Geometry check sheet. Reference: drawing and pictorial views, mm from the part's lowest x, y, z. Coordinates: 2 decimals unless noted, no trailing zeros. Write each loop counter-clockwise with the first axis right and the second up, starting at its lowest first coordinate (ties: lowest second). Pieces come first, ordered by that corner, then holes. Notation, with made-up numbers: (65, 48) -> (98, 48) arc R36 ccw to (98, 82) -> close; hole circle Ø2 at (14.5, 65). An arc over 180 degrees is marked (long way). Use a Markdown table: item, result.
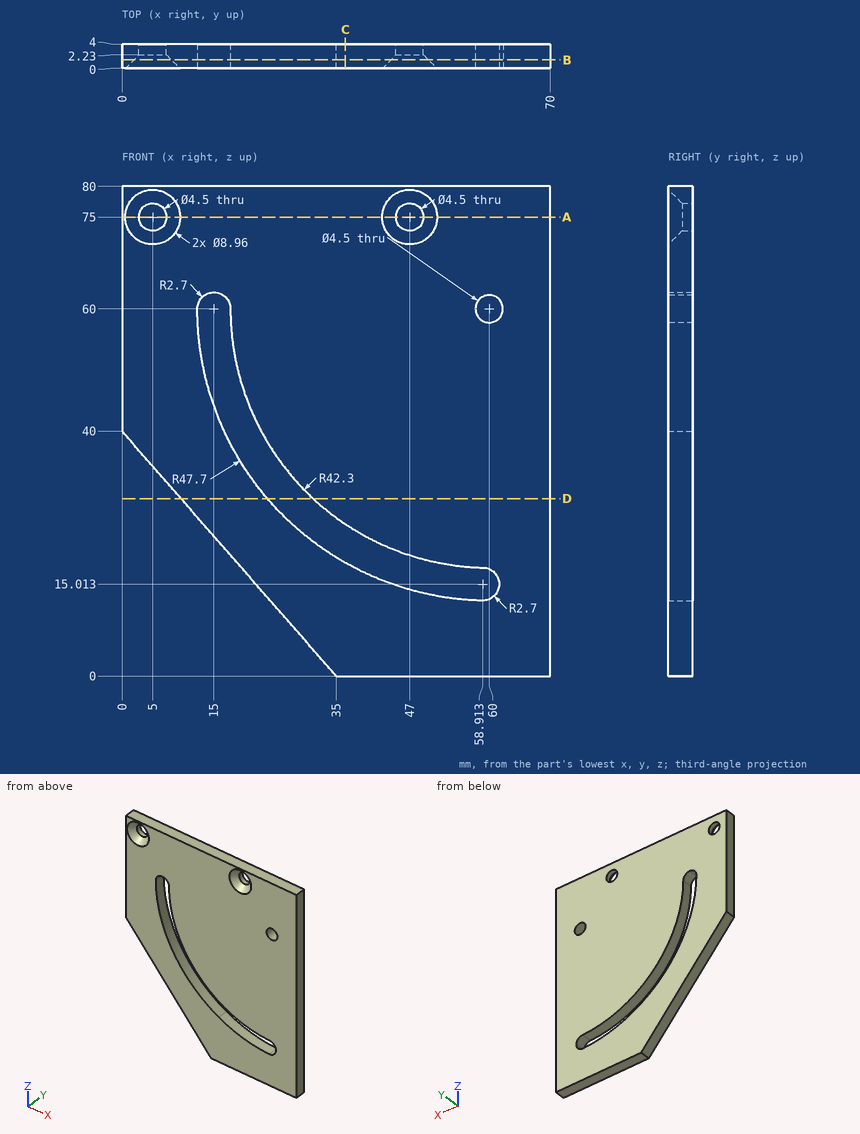
Item 1: Depth check by flat-ended pin: P1, Ø5, axis at x = 5, z = 75, coming from the -Y side; P2, Ø1, axis at x = 16.5, y = 2.5, coming from the -Z side. Enter the tip coordinate at first touch or a pass-through.
Answer block:
| item | result |
|---|---|
| P1 | stops at y = 1.98 |
| P2 | stops at z = 20.57 |
Item 2: Section check A-A on z = 75. Record the boundary of the cut face in (x, y).
Answer block:
| item | result |
|---|---|
| outline | (0, 0) -> (0.52, 0) -> (2.75, 2.23) -> (2.75, 4) -> (0, 4) -> close; (7.25, 2.23) -> (9.48, 0) -> (42.52, 0) -> (44.75, 2.23) -> (44.75, 4) -> (7.25, 4) -> close; (49.25, 2.23) -> (51.48, 0) -> (70, 0) -> (70, 4) -> (49.25, 4) -> close |
Item 3: Section check D-D on z = 29. Record the boundary of the cut face in (x, y) (3 decimals).
Answer block:
| item | result |
|---|---|
| outline | (9.625, 0) -> (23.747, 0) -> (23.747, 4) -> (9.625, 4) -> close; (31.22, 0) -> (70, 0) -> (70, 4) -> (31.22, 4) -> close |
Item 4: Section check B-B on y = 1.4. Count the separate pieces of the cut face and the enclosed holes in it, then the cut area to 3 significant figures.
Answer block:
| item | result |
|---|---|
| separate pieces | 1 |
| enclosed holes | 4 |
| area | 4,430 mm^2 |
Item 5: Section check C-C on x = 36.5. Record the boundary of the cut face in (y, z).
Answer block:
| item | result |
|---|---|
| outline | (0, 0) -> (4, 0) -> (4, 18.49) -> (0, 18.49) -> close; (0, 24.83) -> (4, 24.83) -> (4, 80) -> (0, 80) -> close |
Item 6: Thickness scan on L1, parallel to X at y = 3, z = 75; L2, parallel to Z at x = 47, y = 2.7; L3, parallel to X at y = 1.95, z = 74.5. Record the ranges inside material, lowest first. Write a range as [from, to].
Answer block:
| item | result |
|---|---|
| L1 | x = [0, 2.75], [7.25, 44.75], [49.25, 70] |
| L2 | z = [0, 14.11], [19.75, 72.75], [77.25, 80] |
| L3 | x = [0, 2.52], [7.48, 44.52], [49.48, 70] |
